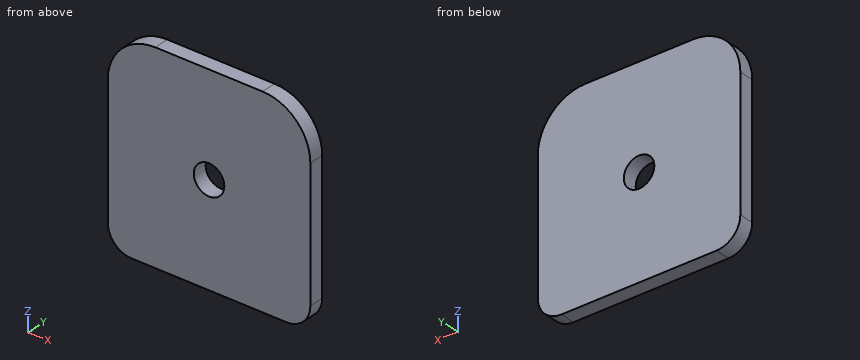
```python
from build123d import *

# Parameters (mm, degrees)
SKETCH1_W           = 85
SKETCH1_H           = 85
BOSS_EXTRUDE1_DEPTH = 6.3
CUT_EXTRUDE1_REACH  = 8.3
SKETCH2_R           = 6.4
FILLET1_R           = 10
FILLET2_R           = 20


with BuildPart() as part:
    # Sketch1 → Boss-Extrude1 (new body)
    with BuildSketch(Plane(origin=(0, 0, 0), x_dir=(1, 0, 0), z_dir=(0, 1, 0))):
        with Locations((42.5, 42.5)):
            Rectangle(SKETCH1_W, SKETCH1_H)
    extrude(amount=BOSS_EXTRUDE1_DEPTH)

    # Sketch2 → Cut-Extrude1 (cut, up to next)
    with BuildSketch(Plane(origin=(0, 6.3, 0), x_dir=(1, 0, 0), z_dir=(0, 1, 0)), mode=Mode.PRIVATE) as cut_extrude1_sk1:
        with Locations((42.5, 42.5)):
            Circle(SKETCH2_R)
    cut_extrude1_tool1 = extrude(cut_extrude1_sk1.sketch, amount=-CUT_EXTRUDE1_REACH, mode=Mode.PRIVATE) & part.part
    add(cut_extrude1_tool1.solids().sort_by_distance((42.5, 6.3, -42.5))[0], mode=Mode.SUBTRACT)

    # Fillet1
    fillet1_edges = [part.edges().sort_by_distance(p)[0] for p in [
        (0, 3.15, -85),
        (85, 3.15, -85),
    ]]
    fillet(fillet1_edges, radius=FILLET1_R)

    # Fillet2
    fillet2_edges = [part.edges().sort_by_distance(p)[0] for p in [
        (85, 3.15, 0),
        (0, 3.15, 0),
    ]]
    fillet(fillet2_edges, radius=FILLET2_R)


solid = part.part
```
Can you work these out from the model? Positions are in its coordinate system, mm. Coordinates: 2 decimals unless noted, no trailing zeros. Order: outer loops, then holes, each group sorted by start corner. A loop starts at its lowest first (then second) coordinate and runs counter-clockwise, first axis right, second up.
1. I'm going to push flat-ended pins straight in: pin 1 (2 mm diameter, centred on x = 27, z = -55.5, fed in from -Y); pin 2 (10 mm diameter, centred on x = 42.5, z = -42.5, fed in from +Y). Where does each tip first touch, or does it pass through?
2. If we section it at A-A (z = -42.5): Please give me the cut outline in (x, y), then the cut area to 3 significant figures.
3. I need wall thicknesses on line 1 (Z direction, x = 42.5, y = 2); line 2 (X direction, y = 4, z = -42.5); line 3 (X direction, y = 2.75, z = -46). Which ranges of each line are inside material? Lowest first, please.
4. If we section it at B-B (y = 2.5): Please give me the cut outline in (x, z).
5. If we section it at C-C (x = 42.5): Please give me the cut outline in (y, z), then the cut area to 3 significant figures.
Entries:
1. pin 1: stops at y = 0
1. pin 2: passes through
2. outline: (0, 0) - (36.1, 0) - (36.1, 6.3) - (0, 6.3) - close; (48.9, 0) - (85, 0) - (85, 6.3) - (48.9, 6.3) - close
2. area: 455 mm2
3. line 1: z = -85 to -48.9, -36.1 to 0
3. line 2: x = 0 to 36.1, 48.9 to 85
3. line 3: x = 0 to 37.14, 47.86 to 85
4. outline: (0, -75) arc R10 ccw to (10, -85) - (75, -85) arc R10 ccw to (85, -75) - (85, -20) arc R20 ccw to (65, 0) - (20, 0) arc R20 ccw to (0, -20) - close; hole circle Ø12.8 at (42.5, -42.5)
5. outline: (0, -85) - (6.3, -85) - (6.3, -48.9) - (0, -48.9) - close; (0, -36.1) - (6.3, -36.1) - (6.3, 0) - (0, 0) - close
5. area: 455 mm2
